Build history of the part. All positions in model axes, mm. A direction names the side the tool comes from. Give positions to 0.01 mm unless a question says otherwise; leave off trailing zeros. Write each loop counter-clockwise with the first axis right and the second up, starting at its lowest first coordinate (ties: lowest second). Pieces come first, ordered by that corner, then holes. Notation, with made-up numbers: (-6, -8.75) -> (28, -8.75) arc R26 cw to (28, 25.25) -> close; hole circle Ø10 at (-16, 66). An arc over 180 degrees is marked (long way). One line per question, with ' | ' between items. Start each with the question number.
(1) Band-saw the part on B-B, the plane x = -87. Give the cut face in (y, z).
(2) Band-saw the part on C-C, the plane y = 51. Give the cut face in (x, z), and give its area (3 significant figures).
(3) Pin check, flat tips, straight feed: P1, Ø1.8, axis at y = 2.5, z = 3.5, coming from the +X side; P2, Ø1.8, axis at y = 51.5, z = 1.5, coming from the -X side; P3, Ø1.5, axis at x = -82.5, z = 4.5, coming from the -Y side. Stop position of each tip, or through.
(4) Tool access for faces 5 (the flat face through (-42, 6, 3)), 6 (the flat face through (-5, 49, 3)), 7 (the flat face through (-116, 6, 3)), 8 (the flat face through (-74, 52, 3)), 9 (the flat face through (-49, 21, 3)): list every direction of +Z, -Z, +X, -X, +Y, -Y with a clear straight run to the whole face (end or side of a thin tool).
(5) Band-saw the part on D-D, the plane z = 2. Count the separate pieces of the cut face and the enclosed holes in it, and give its area (3 significant figures).
(6) Band-saw the part on A-A, the plane y = 23.5. Give the cut face in (x, z).
(7) Pull direction X, two halves, no side cores. Call faces 1 (the flat face through (-37, 3, 3)), 2 (the flat face through (-121, 27, 3)), 3 (the flat face through (-10, 3, 3)), 4 (the flat face through (-5, 6, 3)): released by +X, released by -X, zero draft, split by the parting line, or undercut.
(8) Drill centre lines: probe 1 along X at (y, z) = (26, 5.55); probe 2 along X at (y, z) = (52.5, 2.8); probe 3 along Y at (x, z) = (-76, 0.7). Where is each one in solid material? Low to high. Write a range as from..to.
from build123d import *

# Parameters (mm, degrees)
ESQUISSE1_W             = 121
ESQUISSE1_H             = 55
BOSS_EXTRU_1_DEPTH      = 6
ESQUISSE2_W             = 10
ESQUISSE2_H             = 6
ENL_V_MAT_ENCOCHE_DEPTH = 134.048863204
ESQUISSE3_W             = 24
ESQUISSE3_H             = 12
ENL_V_MAT_EXTRU_2_DEPTH = 6


with BuildPart() as part:
    # Esquisse1 → Boss.-Extru.1 (new body)
    with BuildSketch(Plane.XY):
        with Locations((-60.5, 27.5)):
            Rectangle(ESQUISSE1_W, ESQUISSE1_H)
    extrude(amount=BOSS_EXTRU_1_DEPTH)

    # Esquisse2 → Enlèv. mat encoche (cut, through all)
    with BuildSketch(Plane.XY.offset(6)):
        with Locations((-116, 52)):
            Rectangle(ESQUISSE2_W, ESQUISSE2_H)
        with Locations((-79, 52)):
            Rectangle(ESQUISSE2_W, ESQUISSE2_H)
        with Locations((-42, 52)):
            Rectangle(ESQUISSE2_W, ESQUISSE2_H)
        with Locations((-5, 52)):
            Rectangle(ESQUISSE2_W, ESQUISSE2_H)
        with Locations((-116, 3)):
            Rectangle(ESQUISSE2_W, ESQUISSE2_H)
        with Locations((-79, 3)):
            Rectangle(ESQUISSE2_W, ESQUISSE2_H)
        with Locations((-42, 3)):
            Rectangle(ESQUISSE2_W, ESQUISSE2_H)
        with Locations((-5, 3)):
            Rectangle(ESQUISSE2_W, ESQUISSE2_H)
    extrude(amount=-ENL_V_MAT_ENCOCHE_DEPTH, mode=Mode.SUBTRACT)

    # Esquisse3 → Enlèv. mat.-Extru.2 (cut)
    with BuildSketch(Plane.XY.offset(6)):
        with Locations((-84, 21)):
            Rectangle(ESQUISSE3_W, ESQUISSE3_H)
        with Locations((-37, 21)):
            Rectangle(ESQUISSE3_W, ESQUISSE3_H)
    extrude(amount=-ENL_V_MAT_EXTRU_2_DEPTH, mode=Mode.SUBTRACT)


solid = part.part
Results:
1) outline: (0, 0) -> (15, 0) -> (15, 6) -> (0, 6) -> close; (27, 0) -> (55, 0) -> (55, 6) -> (27, 6) -> close
2) outline: (-111, 0) -> (-84, 0) -> (-84, 6) -> (-111, 6) -> close; (-74, 0) -> (-47, 0) -> (-47, 6) -> (-74, 6) -> close; (-37, 0) -> (-10, 0) -> (-10, 6) -> (-37, 6) -> close | area: 486 mm²
3) P1: stops at x = -10 | P2: stops at x = -111 | P3: stops at y = 6
4) face 5: +Z, -Z, -Y | face 6: +Z, -Z, +X, +Y | face 7: +Z, -Z, -X, -Y | face 8: +Z, -Z, +Y | face 9: +Z, -Z
5) separate pieces: 1 | enclosed holes: 2 | area: 5,600 mm²
6) outline: (-121, 0) -> (-96, 0) -> (-96, 6) -> (-121, 6) -> close; (-72, 0) -> (-49, 0) -> (-49, 6) -> (-72, 6) -> close; (-25, 0) -> (0, 0) -> (0, 6) -> (-25, 6) -> close
7) face 1: undercut | face 2: released by -X | face 3: released by +X | face 4: zero draft
8) probe 1: x = -121..-96, -72..-49, -25..0 | probe 2: x = -111..-84, -74..-47, -37..-10 | probe 3: y = 6..15, 27..49
